```python
from build123d import *

# Parameters (mm, degrees)
F0_W     = 228.6
F0_H     = 50.8
F0_R     = 6.35
F0_R_2   = 11.1125
F1_DEPTH = 19.05


with BuildPart() as f1:
    # F0 (on Front) → F1 (new body)
    with BuildSketch(Plane.XZ):
        with Locations((114.3, 25.4)):
            Rectangle(F0_W, F0_H)
        with Locations((12.7, 25.4)):
            Circle(F0_R, mode=Mode.SUBTRACT)
        with Locations((31.75, 25.4)):
            Circle(F0_R_2, mode=Mode.SUBTRACT)
        with Locations((76.2, 25.4)):
            Circle(F0_R, mode=Mode.SUBTRACT)
        with Locations((120.65, 25.4)):
            Circle(F0_R_2, mode=Mode.SUBTRACT)
        with Locations((139.7, 25.4)):
            Circle(F0_R, mode=Mode.SUBTRACT)
    extrude(amount=F1_DEPTH)


solid = f1.part
```
Source: CAD feature listing. Evaluate the final solid. Frame: model axes, mm. Round coordinates to 2 decimals unless told otherwise and drop trailing zeros. Write each loop counter-clockwise with the first axis right and the second up, starting at its lowest first coordinate (ties: lowest second). Pieces come first, ordered by that corner, then holes. Notation, with made-up numbers: M -27,-28.5 L -7,-28.5 A17 cw -7,-11.5 Z; hole C -8.75,27 d8. An arc over 180 degrees is marked long. Answer as a JSON object with one key per item and string values. Group by question number.
(1) Section query C-C on z = 25.4. Output: boundary loops of the cut face in (x, y).
(2) Section query B-B on y = -13. State how many separate pieces and enclosed holes the cut face has, then the cut area to 3 significant figures.
(3) Ray query, line 1 (X direction, y = -14.5, z = 21); line 2 (Z direction, x = 139.7, y = -7.75); line 3 (X direction, y = -16.5, z = 34). Return the intervals inside material, ascending. Write a range as [from, to].
(4) Section query A-A on x = 31.75. Output: boundary loops of the cut face in (y, z), then the cut area to 3 significant figures.
(5) First-contact query: pin 1 (13.5 mm diameter, centred on x = 31.75, z = 25.4, fed in from -Y). Flat tip, straight axial feed; report the tip coordinate or a pass-through.
(6) Mould query, pull axis Z, two halves, no side actions, for faces 1 (the cylindrical face through (37.724, -9.392, 34.77)), 2 (the flat face through (228.6, -9, 25)), 3 (the flat face through (113, -9, 50.8)), 4 (the cylindrical face through (69.856, -9.392, 25.679)). Classes: +Z half, -Z half, draft (parallel to the pull), parting line (faces both ways), or undercut.
(7) Section query D-D on z = 34.5. Output: boundary loops of the cut face in (x, y), then the cut area to 3 significant figures.
Computed values:
{
 "1": {"outline": "M 0,-19.05 L 6.35,-19.05 L 6.35,0 L 0,0 Z; M 19.05,-19.05 L 20.64,-19.05 L 20.64,0 L 19.05,0 Z; M 42.86,-19.05 L 69.85,-19.05 L 69.85,0 L 42.86,0 Z; M 82.55,-19.05 L 109.54,-19.05 L 109.54,0 L 82.55,0 Z; M 131.76,-19.05 L 133.35,-19.05 L 133.35,0 L 131.76,0 Z; M 146.05,-19.05 L 228.6,-19.05 L 228.6,0 L 146.05,0 Z"},
 "2": {"separate pieces": "1", "enclosed holes": "5", "area": "10,500 mm^2"},
 "3": {"line 1": "[0, 8.12], [17.28, 21.55], [41.95, 71.62], [80.78, 110.45], [130.85, 135.12], [144.28, 228.6]", "line 2": "[0, 19.05], [31.75, 50.8]", "line 3": "[0, 24.71], [38.79, 113.61], [127.69, 228.6]"},
 "4": {"outline": "M -19.05,0 L 0,0 L 0,14.29 L -19.05,14.29 Z; M -19.05,36.51 L 0,36.51 L 0,50.8 L -19.05,50.8 Z", "area": "544 mm^2"},
 "5": {"pin 1": "through"},
 "6": {"face 1": "undercut", "face 2": "draft", "face 3": "+Z half", "face 4": "undercut"},
 "7": {"outline": "M 0,-19.05 L 25.37,-19.05 L 25.37,0 L 0,0 Z; M 38.13,-19.05 L 114.27,-19.05 L 114.27,0 L 38.13,0 Z; M 127.03,-19.05 L 228.6,-19.05 L 228.6,0 L 127.03,0 Z", "area": "3,870 mm^2"}
}
